Answer from the drawing. Dimensions are ordinates in mm from the lowest x, y and z of the part. A direction names the side the tool comes from. Coordinates: 2 decimals unless noted, no trailing zeros. Write each loop counter-clockwise with the first axis right and the second up, starting at its lowest first coordinate (ties: lowest second). Pieces come first, ordered by that corner, then holes.
1) The part is cut by section B-B (x = 1.7). Determine the outline of the cut face in (y, z), then the cut area to 3 significant figures.
2) The part is cut by section A-A (z = 6). Determine the outline of the cut face in (x, y), then the cut area to 3 significant figures.
3) Which of the six approach directions +Z, -Z, +X, -X, +Y, -Y give full straight-line access (tool end or side, diameter ignored) to the marked faces 4 and 5?
4) Each of these flat-tipped pins is pushed along its axis until it touches: pin 1 Ø1.9 at (x, z) = (2.5, 6) entering from +Y; pin 2 Ø2.5 at (x, y) = (2, 14) entering from +Z. Where does it stop, or does it pass through?
5) The part is cut by section C-C (z = 7.25). Determine the outline of the cut face in (x, y).
6) Determine the mould class of the marked faces 1, 2 and 3 for opening direction X: +X half, -X half, draft (parallel to the pull), parting line (faces both ways), or undercut.
7) The part is cut by section D-D (y = 20). Determine the outline of the cut face in (x, z), then the cut area to 3 significant figures.
8) Find the intervals of material crossed by line 1 (Z direction, x = 2.5, y = 29.9); line 2 (X direction, y = 29.65, z = 6); line 3 (Y direction, x = 2.7, z = 3), in increasing order.
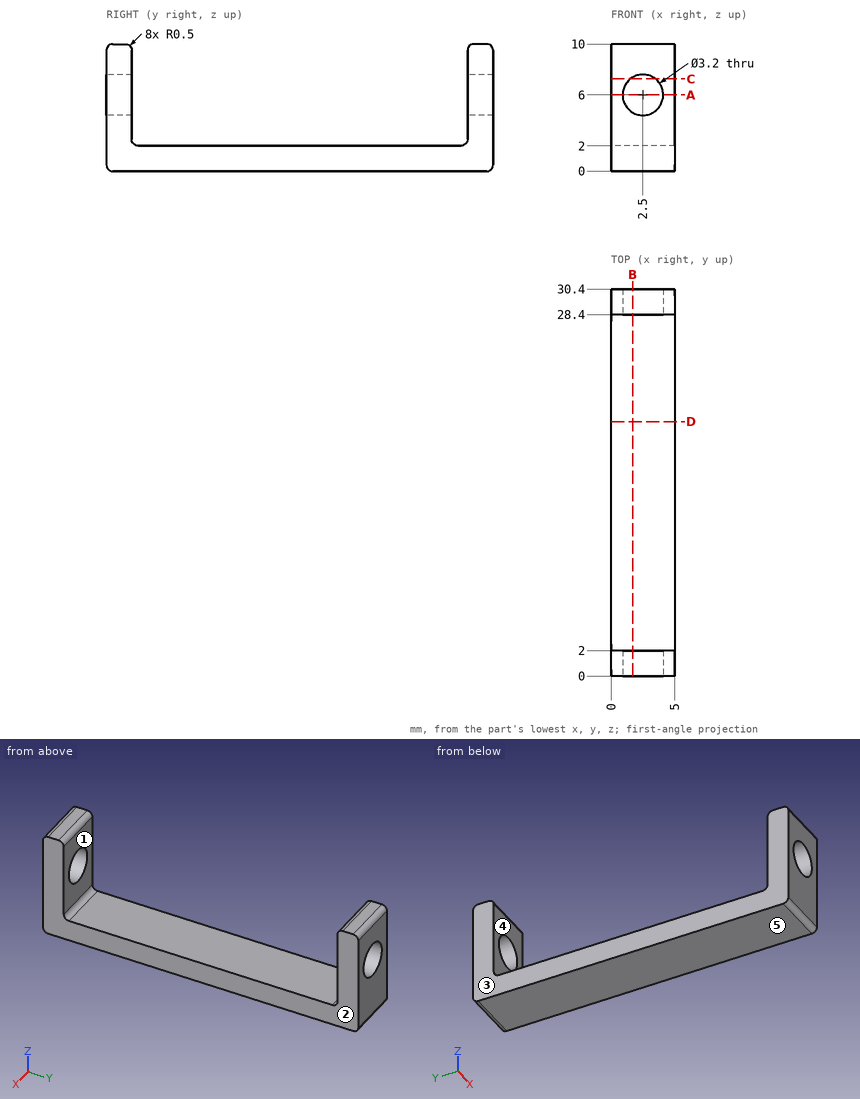
Reported:
1. outline: (0, 0.5) arc R0.5 ccw to (0.5, 0) - (29.9, 0) arc R0.5 ccw to (30.4, 0.5) - (30.4, 4.61) - (28.4, 4.61) - (28.4, 2.5) arc R0.5 cw to (27.9, 2) - (2.5, 2) arc R0.5 cw to (2, 2.5) - (2, 4.61) - (0, 4.61) - close; (0, 7.39) - (2, 7.39) - (2, 9.5) arc R0.5 ccw to (1.5, 10) - (0.5, 10) arc R0.5 ccw to (0, 9.5) - close; (28.4, 7.39) - (30.4, 7.39) - (30.4, 9.5) arc R0.5 ccw to (29.9, 10) - (28.9, 10) arc R0.5 ccw to (28.4, 9.5) - close
1. area: 81.5 mm2
2. outline: (0, 0) - (0.9, 0) - (0.9, 2) - (0, 2) - close; (0, 28.4) - (0.9, 28.4) - (0.9, 30.4) - (0, 30.4) - close; (4.1, 0) - (5, 0) - (5, 2) - (4.1, 2) - close; (4.1, 28.4) - (5, 28.4) - (5, 30.4) - (4.1, 30.4) - close
2. area: 7.20 mm2
3. face 4: +Z, +X, -X
3. face 5: -Z, +X, -X, +Y, -Y
4. pin 1: passes through
4. pin 2: stops at z = 2
5. outline: (0, 0) - (1.5, 0) - (1.5, 2) - (0, 2) - close; (0, 28.4) - (1.5, 28.4) - (1.5, 30.4) - (0, 30.4) - close; (3.5, 0) - (5, 0) - (5, 2) - (3.5, 2) - close; (3.5, 28.4) - (5, 28.4) - (5, 30.4) - (3.5, 30.4) - close
6. face 1: draft
6. face 2: +X half
6. face 3: -X half
7. outline: (0, 0) - (5, 0) - (5, 2) - (0, 2) - close
7. area: 10.0 mm2
8. line 1: z = 0 to 4.4, 7.6 to 10
8. line 2: x = 0 to 0.9, 4.1 to 5
8. line 3: y = 0 to 2, 28.4 to 30.4
